Check sheet for the modelled part. Datum: model origin and axes. Units: mm. Give positions to 0.01 mm unless a question says otherwise; leave off trailing zeros. Loops run counter-clockwise (first coordinate to the right, second up) from the corner with the lowest first, then second, coordinate; pieces in that order, holes last. Notation, with made-up numbers: (-30, 86.5) - (-15, 86.5) arc R22 ccw to (-15, 124.5) - close; hole circle Ø4 at (35, -35.75). An arc over 180 degrees is marked (long way). Use one line per item in the form item = value.
from build123d import *

# Parameters (mm, degrees)
SKETCH_1_R      = 1.75
EXTRUDE_1_DEPTH = 5
FILLET_1_R      = 2
FILLET_2_R      = 2
FILLET_3_R      = 2


with BuildPart() as part:
    # 草图1 → 凸台-拉伸1 (new body)
    with BuildSketch(Plane(origin=(0, 0, 0), x_dir=(1, 0, 0), z_dir=(0, 1, 0))):
        Polygon((-10, 10), (-10, -10), (10, -10), (30, -10), (30, 10), (10, 10), align=None)
        with Locations(Location((0, 0, 0), (0, 0, 270))):
            Circle(SKETCH_1_R, mode=Mode.SUBTRACT)
        with Locations(Location((20, 0, 0), (0, 0, 270))):
            Circle(SKETCH_1_R, mode=Mode.SUBTRACT)
    extrude(amount=EXTRUDE_1_DEPTH)

    # 圆角1
    fillet_1_edges = [part.edges().sort_by_distance(p)[0] for p in [
        (30, 2.5, 10),
        (30, 2.5, -10),
    ]]
    fillet(fillet_1_edges, radius=FILLET_1_R)

    # 圆角2
    fillet_2_edges = [part.edges().sort_by_distance(p)[0] for p in [
        (-10, 2.5, 10),
    ]]
    fillet(fillet_2_edges, radius=FILLET_2_R)

    # 圆角3
    fillet_3_edges = [part.edges().sort_by_distance(p)[0] for p in [
        (-10, 2.5, -10),
    ]]
    fillet(fillet_3_edges, radius=FILLET_3_R)


solid = part.part
Item 1: Mould release check, pull along X, two halves, no side actions. Record for faces 1 (the face through (-1.71, 2.46, -0.38)), 2 (the face through (-9.43, 2.54, -9.4)), 3 (the face through (29.4, 2.54, 9.43)): released by +X, released by -X, zero draft, split by the parting line, or undercut.
Answer block:
face_1 = undercut
face_2 = released by -X
face_3 = released by +X
Item 2: Thickness scan on L1, parallel to X at y = 3.45, z = 0; L2, parallel to X at y = 1.4, z = -1.25; L3, parallel to X at y = 2.4, z = 8.75. Record the ranges inside material, lowest first.
Answer block:
L1 = -10 to -1.75, 1.75 to 18.25, 21.75 to 30
L2 = -10 to -1.22, 1.22 to 18.78, 21.22 to 30
L3 = -9.85 to 29.85
Item 3: Section check A-A on z = 0. Record the boundary of the cut face in (x, y).
Answer block:
outline = (-10, 0) - (-1.75, 0) - (-1.75, 5) - (-10, 5) - close; (1.75, 0) - (18.25, 0) - (18.25, 5) - (1.75, 5) - close; (21.75, 0) - (30, 0) - (30, 5) - (21.75, 5) - close
Item 4: Section check B-B on x = 20. Record the boundary of the cut face in (y, z), then the cut area to 3 significant figures.
Answer block:
outline = (0, -10) - (5, -10) - (5, -1.75) - (0, -1.75) - close; (0, 1.75) - (5, 1.75) - (5, 10) - (0, 10) - close
area = 82.5 mm2
Item 5: Gauge pin test, flat end, axial feed: P1, Ø4, axis at x = 0, z = 0, coming from the +Y side. Record the tip position at first contact, or that the pin passes through.
Answer block:
P1 = 5
Item 6: Section check C-C on y = 2.5. Record the boundary of the cut face in (x, z).
Answer block:
outline = (-10, -8) arc R2 ccw to (-8, -10) - (28, -10) arc R2 ccw to (30, -8) - (30, 8) arc R2 ccw to (28, 10) - (-8, 10) arc R2 ccw to (-10, 8) - close; hole circle Ø3.5 at (0, 0); hole circle Ø3.5 at (20, 0)
